from build123d import *

# Parameters (mm, degrees)
SKETCH1_R           = 1.75
BOSS_EXTRUDE3_DEPTH = 2
BOSS_EXTRUDE4_DEPTH = 20
BOSS_EXTRUDE5_DEPTH = 4


with BuildPart() as part:
    # Sketch1 → Boss-Extrude3 (new body)
    # profile 1 of 3: a face of its own
    with BuildSketch(Plane(origin=(0, 0, 0), x_dir=(1, 0, 0), z_dir=(0, 1, 0))):
        with BuildLine():
            Line((0.004495957, 4.5), (-3.991008085, 4.5))
            ThreePointArc((-3.991008085, 4.5), (-7.240580672, 0), (-3.991008085, -4.5))
            Line((-3.991008085, -4.5), (0.004495957, -4.5))
            ThreePointArc((0.004495957, -4.5), (2.65, 0), (0.004495957, 4.5))
        make_face()
        with Locations(Location((-2.5, 0, 0), (0, 0, 270))):
            Circle(SKETCH1_R, mode=Mode.SUBTRACT)
    # profile 2 of 3: a face of its own
    with BuildSketch(Plane(origin=(0, 0, 0), x_dir=(1, 0, 0), z_dir=(0, 1, 0))):
        with BuildLine():
            Line((4, 4.5), (0.004495957, 4.5))
            ThreePointArc((0.004495957, 4.5), (2.65, 0), (0.004495957, -4.5))
            Line((0.004495957, -4.5), (4, -4.5))
            Line((4, -4.5), (4, 3.5))
            ThreePointArc((4, 3.5), (4.292893219, 4.207106781), (5, 4.5))
            Line((5, 4.5), (4, 4.5))
        make_face()
    # profile 3 of 3: a face of its own
    with BuildSketch(Plane(origin=(0, 0, 0), x_dir=(1, 0, 0), z_dir=(0, 1, 0))):
        with BuildLine():
            Line((7, 4.5), (5, 4.5))
            ThreePointArc((5, 4.5), (4.292893219, 4.207106781), (4, 3.5))
            Line((4, 3.5), (4, -4.5))
            Line((4, -4.5), (7, -4.5))
            Line((7, -4.5), (7, 4.5))
        make_face()
    extrude(amount=BOSS_EXTRUDE3_DEPTH)

    # Sketch1_3 → Boss-Extrude4 (add)
    with BuildSketch(Plane(origin=(0, 0, 0), x_dir=(1, 0, 0), z_dir=(0, 1, 0))):
        with BuildLine():
            ThreePointArc((0.004495957, 4.5), (2.65, 0), (0.004495957, -4.5))
            Line((0.004495957, -4.5), (7, -4.5))
            Line((7, -4.5), (7, 4.5))
            Line((7, 4.5), (0.004495957, 4.5))
        make_face()
    extrude(amount=-BOSS_EXTRUDE4_DEPTH)

    # Sketch1_5 → Boss-Extrude5 (add)
    with BuildSketch(Plane(origin=(0, 0, 0), x_dir=(1, 0, 0), z_dir=(0, 1, 0))):
        with BuildLine():
            Line((7, 4.5), (5, 4.5))
            ThreePointArc((5, 4.5), (4.292893219, 4.207106781), (4, 3.5))
            Line((4, 3.5), (4, -4.5))
            Line((4, -4.5), (7, -4.5))
            Line((7, -4.5), (7, 4.5))
        make_face()
    extrude(amount=BOSS_EXTRUDE5_DEPTH)

    # Mirror1: part across plane


with BuildPart() as part_1:
    add(part.part)
    add(part.part.mirror(Plane.ZX.offset(-20)))


solid = part_1.part
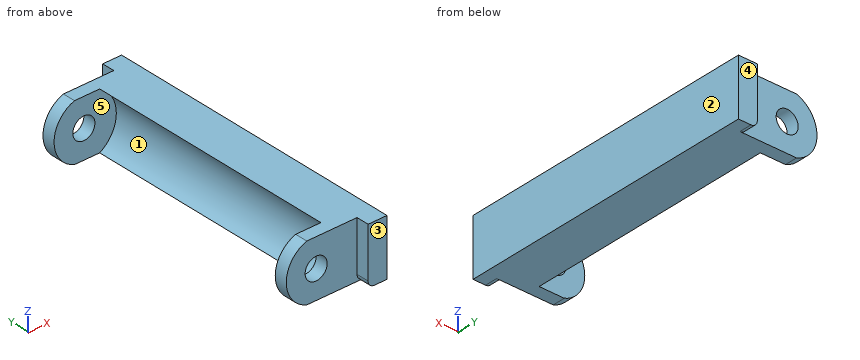
Input: part model. Units: mm. Frame: model coordinates. Face numbers are marked on the shaded views. A direction names the side the tool comes from. Coordinates: 2 decimals unless noted, no trailing zeros. Order: outer loops, then holes, each group sorted by start corner. A loop starts at its lowest first (then second) coordinate and runs counter-clockwise, first axis right, second up. Notation, with made-up numbers: M 23.25,-20 L 50.25,-20 A30 ccw 50.25,6 Z; hole C 83.25,9.5 d1. An arc over 180 degrees is marked long. Answer in a Markdown table with one row per item.
(1) Material intervals for line 1 (Y direction, x = -4.5, z = -2.75); line 2 (X direction, y = 1.35, z = 0); line 3 (X direction, y = -7, z = -2), sorted ascending. Write a range as [from, to].
Numbers:
| item | result |
|---|---|
| line 1 | y = [-42, -40], [0, 2] |
| line 2 | x = [-7.24, -4.25], [-0.75, 7] |
| line 3 | x = [2.25, 7] |
(2) Section query D-D, the plane x = 3.25. Output: boundary loops of the cut face in (y, z).
Numbers:
| item | result |
|---|---|
| outline | M -42,-4.5 L 2,-4.5 L 2,4.5 L -42,4.5 Z |
(3) Contact query for flat-ended pins moving along their axis: pin 1 Ø4.5 at (x, z) = (-4, -2) entering from -Y; pin 2 Ø2.5 at (x, z) = (-1, -1.5) entering from +Y; pin 3 Ø0.6 at (y, z) = (-43, 1) entering from -X; pin 4 Ø3 at (x, z) = (-2.5, 0) entering from -Y. Output: stop coordinate, or through.
Numbers:
| item | result |
|---|---|
| pin 1 | stops at y = -42 |
| pin 2 | stops at y = 2 |
| pin 3 | stops at x = 4 |
| pin 4 | passes through |
(4) Access query for the marked faces 4 and 5. Directions: +Z, -Z, +X, -X, +Y, -Y. A direction counts if a zero-diameter tool reaches every point of the face in a straight line with its end or side. Return the directions, or none.
Numbers:
| item | result |
|---|---|
| face 4 | +Z, -Z, +X, -X, +Y |
| face 5 | -X |
(5) Section query C-C, the plane y = -31.5. Output: boundary loops of the cut face in (x, z), plus the area to 3 significant figures.
Numbers:
| item | result |
|---|---|
| outline | M 0,-4.5 L 7,-4.5 L 7,4.5 L 0,4.5 A5.15 cw Z |
| area | 46.0 mm^2 |
(6) Draft query along Y for the marked faces 1, 2 and 3. Return one class per face: pulls with the +Y half, pulls with the -Y half, needs draft (parallel to the pull), parting line crosses it, or undercut.
Numbers:
| item | result |
|---|---|
| face 1 | undercut |
| face 2 | needs draft |
| face 3 | pulls with the -Y half |
(7) Section query A-A, the plane z = -0.25. Output: boundary loops of the cut face in (x, y), plus the area to 3 significant figures.
Numbers:
| item | result |
|---|---|
| outline | M -7.23,-42 L -4.23,-42 L -4.23,-40 L -7.23,-40 Z; M -7.23,0 L -4.23,0 L -4.23,2 L -7.23,2 Z; M -0.77,-42 L 4,-42 L 4,-44 L 7,-44 L 7,4 L 4,4 L 4,2 L -0.77,2 L -0.77,0 L 2.64,0 L 2.64,-40 L -0.77,-40 Z |
| area | 229 mm^2 |
(8) Section query B-B, the plane x = -2.5. Output: boundary loops of the cut face in (y, z), plus the area to 3 significant figures.
Numbers:
| item | result |
|---|---|
| outline | M -42,-4.5 L -40,-4.5 L -40,-1.75 L -42,-1.75 Z; M -42,1.75 L -40,1.75 L -40,4.5 L -42,4.5 Z; M 0,-4.5 L 2,-4.5 L 2,-1.75 L 0,-1.75 Z; M 0,1.75 L 2,1.75 L 2,4.5 L 0,4.5 Z |
| area | 22.0 mm^2 |
